```python
from build123d import *

# Parameters (mm, degrees)
SKETCH002_R      = 1.6
PAD002_DEPTH     = 10
PAD001_DEPTH     = 2.5
CLONE_ROLL_ANGLE = 180
SKETCH003_R      = 11.5
SKETCH003_R_2    = 10
PAD003_DEPTH     = 1.5
PAD_DEPTH        = 12


with BuildPart() as pad002:
    # Sketch002 → Pad002 (new body)
    with BuildSketch(Plane.XZ.offset(6)):
        with Locations((-15, 7)):
            Circle(SKETCH002_R)
        with Locations((0, -7)):
            Circle(SKETCH002_R)
        with Locations((15, 7)):
            Circle(SKETCH002_R)
        with Locations((-15, -7)):
            Circle(SKETCH002_R)
        with Locations((0, 7)):
            Circle(SKETCH002_R)
        with Locations((15, -7)):
            Circle(SKETCH002_R)
    extrude(amount=PAD002_DEPTH)


with BuildPart() as pad001:
    # Sketch001 → Pad001 (new body)
    with BuildSketch(Plane.XZ.offset(6)):
        Polygon((-12.185417, 5.375), (-12.185417, 8.625), (-15, 10.25), (-17.814583, 8.625), (-17.814583, 5.375), (-15, 3.75), align=None)
        Polygon((2.814583, -8.625), (2.814583, -5.375), (0, -3.75), (-2.814583, -5.375), (-2.814583, -8.625), (0, -10.25), align=None)
        Polygon((17.814583, 5.375), (17.814583, 8.625), (15, 10.25), (12.185417, 8.625), (12.185417, 5.375), (15, 3.75), align=None)
    extrude(amount=PAD001_DEPTH)


with BuildPart() as fusion:
    # Clone base: copy of Pad001
    add(pad001.part)


with BuildPart() as fusion_1:
    # Clone roll: moved
    add(fusion.part.rotate(Axis((0, 0, 0), (1, 0, 0)), CLONE_ROLL_ANGLE))


with BuildPart() as fusion_2:
    # Clone placement: moved
    add(fusion_1.part.moved(Location((0, -17, 0))))

    # Fusion: union Pad002, Pad001
    add(pad002.part)
    add(pad001.part)


with BuildPart() as pad003:
    # Sketch003 → Pad003 (new body, symmetric)
    with BuildSketch(Plane.XY):
        with Locations((-30, 0)):
            Circle(SKETCH003_R)
        with Locations((-30, 0)):
            Circle(SKETCH003_R_2, mode=Mode.SUBTRACT)
    extrude(amount=PAD003_DEPTH, both=True)


with BuildPart() as clone_of_pad003:
    # Clone002 base: copy of Pad003
    add(pad003.part)


with BuildPart() as clone_of_pad003_1:
    # Clone002 placement: moved
    add(clone_of_pad003.part.moved(Location((0, 0, -7))))


with BuildPart() as fusion002:
    # Clone001 base: copy of Pad003
    add(pad003.part)


with BuildPart() as fusion002_1:
    # Clone001 placement: moved
    add(fusion002.part.moved(Location((0, 0, 7))))

    # Fusion002: union Clone of Pad003
    add(clone_of_pad003_1.part)


with BuildPart() as cut:
    # Sketch → Pad (new body, symmetric)
    with BuildSketch(Plane.XY):
        with BuildLine():
            ThreePointArc((-37.047695, 2.565151), (-30, -7.5), (-22.952305, 2.565151))
            Line((-22.952305, 2.565151), (-20.133227, 3.591212))
            ThreePointArc((-19.5, 0), (-19.659519, 1.823306), (-20.133227, 3.591212))
            Line((-19.5, 0), (-19.5, -6))
            Line((-19.5, -6), (0, -6))
            Line((0, -6), (0, -11))
            Line((0, -11), (-28.266296, -11))
            ThreePointArc((-35.591373, -8.887438), (-32.078109, -10.461312), (-28.266296, -11))
            ThreePointArc((-39.866773, 3.591212), (-39.933163, -3.403273), (-35.591373, -8.887438))
            Line((-37.047695, 2.565151), (-39.866773, 3.591212))
        make_face()
    extrude(amount=PAD_DEPTH, both=True)

    # Cut: cut Fusion002
    add(fusion002_1.part, mode=Mode.SUBTRACT)


with BuildPart() as cut001:
    # Part__Mirroring: instance of Cut
    add(cut.part.mirror(Plane(origin=(0, 0, 0), x_dir=(0, -1, 0), z_dir=(1, 0, 0))))

    # Fusion003: union Cut
    add(cut.part)

    # Cut001: cut Fusion
    add(fusion_2.part, mode=Mode.SUBTRACT)


solid = cut001.part
```
Geometry: final body of the model. Coordinates: model frame, mm. A direction names the side the tool comes from. Round coordinates to 2 decimals unless told otherwise and drop trailing zeros. Loops run counter-clockwise (first coordinate to the right, second up) from the corner with the lowest first, then second, coordinate; pieces in that order, holes last. Notation, with made-up numbers: (30, -15) -> (48, -15) arc R11 ccw to (48, 3) -> close; hole circle Ø1 at (13, 59.25). An arc over 180 degrees is marked (long way). Use one line per item in the form item = value. Start each with the question number.
1) First-contact query: P1, Ø6, axis at x = -15.5, z = 8.5, coming from the +Y side; P2, Ø2, axis at y = -8, z = 7, coming from the +X side; P3, Ø2, axis at y = -4.5, z = -2.5, coming from the +X side. Flat tips, straight axial feed; report the tip coordinate or a pass-through.
2) Section A-A on z = -0.5. Output: boundary loops of the cut face in (x, y), then the cut area to 3 significant figures.
3) Section C-C on y = -3.5. Give the number of separate pieces and of enclosed holes in the cut face, then the cut area to 3 significant figures.
4) Line query: L1, parallel to Z at x = 15, y = -7.65; L2, parallel to Z at x = 15, y = -9.05; L3, parallel to X at y = -4, z = 8. Output: solid intervals per line, ascending.
5) Access query for faces 4 (the flat face through (-17.815, -10, -7)), 5 (the flat face through (21.56, 3.07, 0.17)), 6 (the cylindrical face through (-39.965, -3.309, 10.274)), 7 (the flat face through (16.388, -7.232, 4.551)), 8 (the cylindrical face through (-22.44, -8.666, 7.021)). Directions: +Z, -Z, +X, -X, +Y, -Y. A direction counts if a zero-diameter tool reaches every point of the face in a straight line with its end or side. Return the directions, or none.
6) Draft query along X for faces 1 (the cylindrical face through (32.13, -10.446, -10.226)), 2 (the flat face through (1.388, -9.767, 9.449)), 3 (the cylindrical face through (-32.13, -10.446, -10.226)). Return one class per face: released by +X, released by -X, zero draft, split by the parting line, or undercut.
7) Section B-B on x = -25.5. Output: boundary loops of the cut face in (y, z).
Response:
q1.P1 = -6
q1.P2 = 37.14
q1.P3 = 39.9
q2.outline = (-39.87, 3.59) arc R10.5 ccw to (-35.59, -8.89) arc R13.76 ccw to (-28.27, -11) -> (28.27, -11) arc R13.76 ccw to (35.59, -8.89) arc R10.5 ccw to (39.87, 3.59) -> (37.05, 2.57) arc R7.5 cw (long way) to (22.95, 2.57) -> (20.13, 3.59) arc R10.5 ccw to (19.5, 0) -> (19.5, -6) -> (-19.5, -6) -> (-19.5, 0) arc R10.5 ccw to (-20.13, 3.59) -> (-22.95, 2.57) arc R7.5 cw (long way) to (-37.05, 2.57) -> close
q2.area = 462 mm^2
q3.separate_pieces = 4
q3.enclosed_holes = 0
q3.area = 322 mm^2
q4.L1 = -12 to -8.6, -5.4 to 3.75, 10.25 to 12
q4.L2 = -12 to -10.25, -3.75 to 5.4, 8.6 to 12
q4.L3 = -39.17 to -36.34, -23.66 to -20.83, 20.83 to 23.66, 36.34 to 39.17
q5.face_4 = -Y
q5.face_5 = +Z, -Z, +Y
q5.face_6 = +Z, -Z, -X
q5.face_7 = +Y
q5.face_8 = none
q6.face_1 = released by +X
q6.face_2 = undercut
q6.face_3 = released by -X
q7.outline = (-11, -12) -> (-6, -12) -> (-6, 12) -> (-11, 12) -> close; hole (-10.58, -8.5) -> (-8.93, -8.5) -> (-8.93, -5.5) -> (-10.58, -5.5) -> close; hole (-10.58, 5.5) -> (-8.93, 5.5) -> (-8.93, 8.5) -> (-10.58, 8.5) -> close
